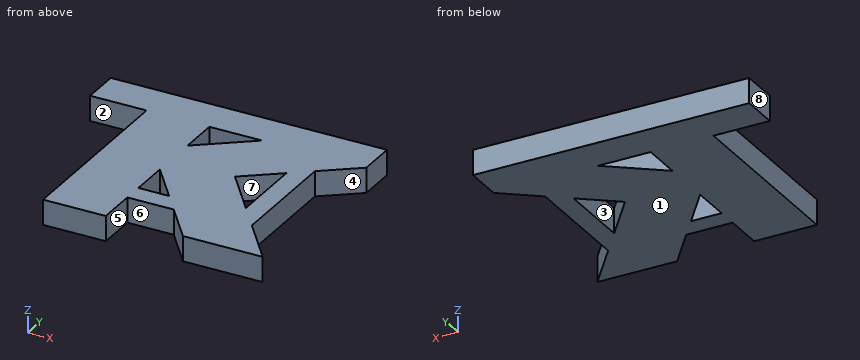
```python
from build123d import *

# Parameters (mm, degrees)
BOSS_EXTRUDE1_DEPTH = 10


with BuildPart() as part:
    # Sketch1 → Boss-Extrude1 (new body)
    # profile 1 of 3: a face of its own
    with BuildSketch(Plane.XY):
        Polygon((87.5, 75), (87.5, 90), (-22.5, 90), (-22.5, 75), (0, 75), (0, 0), (25, 0), (25, 39.184229931), (55.729251038, 0), (87.5, 0), (50.538942191, 47.130682941), align=None)
        Polygon((45.975310969, 75), (25, 59.184229931), (25, 75), align=None, mode=Mode.SUBTRACT)
    # profile 2 of 3: a face of its own
    with BuildSketch(Plane.XY):
        Polygon((25, 23.592114965), (25, 15.592114965), (43.501525347, 15.592114965), (37.22772569, 23.592114965), align=None)
    # profile 3 of 3: a face of its own
    with BuildSketch(Plane.XY):
        Polygon((73.019471096, 18.464764189), (73.019471096, 64.081415004), (65.019471096, 58.049267937), (65.019471096, 28.665918752), align=None)
    extrude(amount=BOSS_EXTRUDE1_DEPTH)


solid = part.part
```
Read the model definition and answer for the solid it produces. Units are mm, in the model's axes. Face numbers are marked on the shaded views. A direction names the side the tool comes from. Coordinates: 2 decimals unless noted, no trailing zeros. Loops run counter-clockwise (first coordinate to the right, second up) from the corner with the lowest first, then second, coordinate; pieces in that order, holes last. Notation, with made-up numbers: (36, 22) - (72, 22) arc R14 ccw to (72, 38) - close; hole circle Ø7 at (67.5, 21). An arc over 180 degrees is marked (long way). Answer in a Markdown table with one row per item.
1. Which of the six approach directions +Z, -Z, +X, -X, +Y, -Y give full straight-line access (tool end or side, diameter ignored) to the marked faces 1, 2, 3, 4 and 5?
Conclusion:
| item | result |
|---|---|
| face 1 | -Z, +X, -X, +Y, -Y |
| face 2 | +Z, -Z, -X, -Y |
| face 3 | +Z, -Z |
| face 4 | +Z, -Z, +X |
| face 5 | +Z, -Z, -Y |
2. Straight lines are drawn through the part: line 1 (X direction, y = 34, z = 5); line 2 (X direction, y = 31, z = 2.5); line 3 (X direction, y = 26.5, z = 3.5). For each, find the intervals that lie inside material, in ascending order.
Conclusion:
| item | result |
|---|---|
| line 1 | x = 0 to 25, 29.07 to 60.84, 65.02 to 73.02 |
| line 2 | x = 0 to 25, 31.42 to 63.19, 65.02 to 73.02 |
| line 3 | x = 0 to 25, 34.95 to 73.02 |
3. Determine the mould class of the marked faces 6, 7 and 8 for opening direction Y: +Y half, -Y half, draft (parallel to the pull), parting line (faces both ways), or undercut.
Conclusion:
| item | result |
|---|---|
| face 6 | -Y half |
| face 7 | undercut |
| face 8 | draft |
4. Find section D-D, the plane x = 57. Write down the section's boundary in (y, z), then the cut area to 3 significant figures.
Conclusion:
| item | result |
|---|---|
| outline | (0, 0) - (38.89, 0) - (38.89, 10) - (0, 10) - close; (52, 0) - (90, 0) - (90, 10) - (52, 10) - close |
| area | 769 mm² |
5. Find section B-B, the plane x = 31. Write down the section's boundary in (y, z).
Conclusion:
| item | result |
|---|---|
| outline | (15.59, 0) - (23.59, 0) - (23.59, 10) - (15.59, 10) - close; (31.53, 0) - (63.71, 0) - (63.71, 10) - (31.53, 10) - close; (75, 0) - (90, 0) - (90, 10) - (75, 10) - close |
6. Find section C-C, the plane y = 56. Write down the section's boundary in (x, z).
Conclusion:
| item | result |
|---|---|
| outline | (0, 0) - (62.3, 0) - (62.3, 10) - (0, 10) - close; (65.02, 0) - (73.02, 0) - (73.02, 10) - (65.02, 10) - close |
7. Find section A-A, the plane z = 8. Write down the section's boundary in (x, y).
Conclusion:
| item | result |
|---|---|
| outline | (-22.5, 75) - (0, 75) - (0, 0) - (25, 0) - (25, 15.59) - (43.5, 15.59) - (55.73, 0) - (87.5, 0) - (73.02, 18.46) - (73.02, 64.08) - (87.5, 75) - (87.5, 90) - (-22.5, 90) - close; hole (25, 23.59) - (37.23, 23.59) - (25, 39.18) - close; hole (25, 59.18) - (45.98, 75) - (25, 75) - close; hole (50.54, 47.13) - (65.02, 28.67) - (65.02, 58.05) - close |
8. Given pin 1 (1 mm diameter, centred on x = 28, z = 5, fed in from -Y); pin 2 (5 mm diameter, centred on x = -6, z = 3.5, fed in from -Y); pin 3 (6 mm diameter, centred on y = 14, z = 8.5, fed in from -X), each flat-ended and moving along its own axis, determine where each tip first touches the part or whether it passes through.
Conclusion:
| item | result |
|---|---|
| pin 1 | stops at y = 15.59 |
| pin 2 | stops at y = 75 |
| pin 3 | stops at x = 0 |
